Here's the drawing with two shaded views (mm, measured from the low corner). I have some questions. A direction names the side the tool comes from. Round coordinates to 2 decimals unless told otherwise and drop trailing zeros. Loops run counter-clockwise (first coordinate to the right, second up) from the corner with the lowest first, then second, coordinate; pieces in that order, holes last.
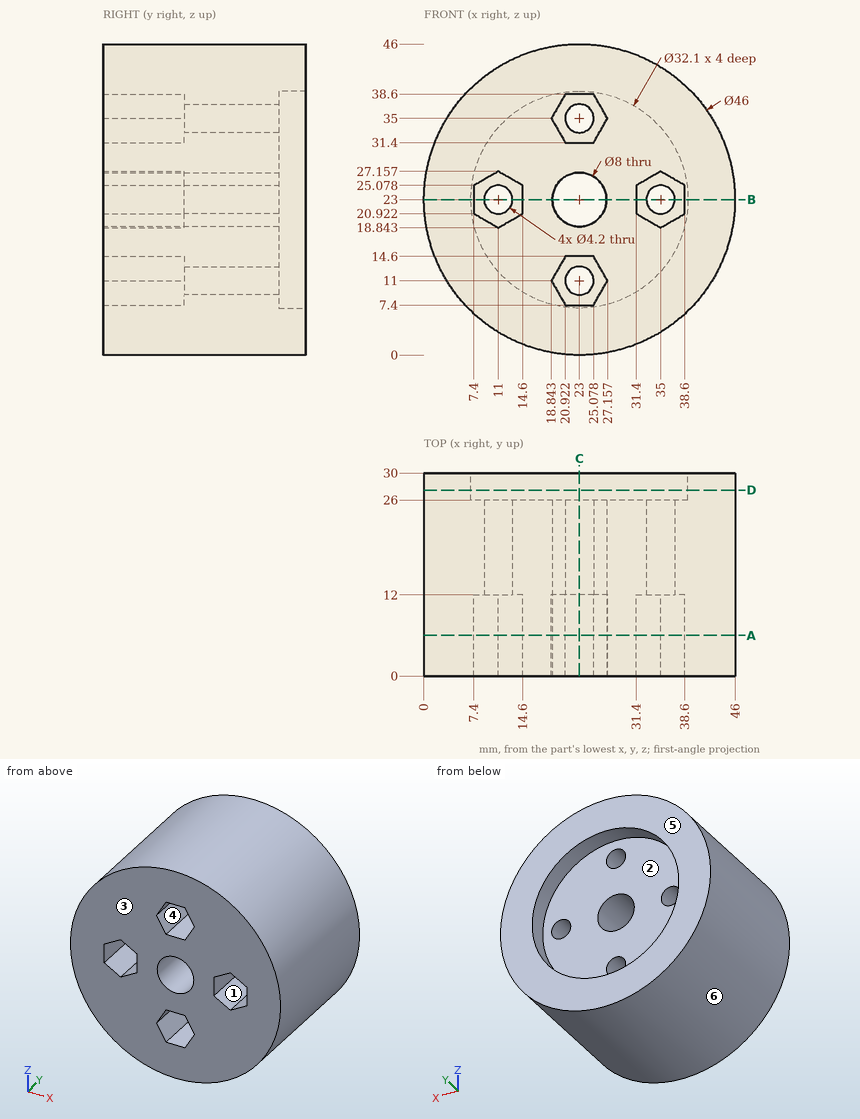
Item 1: If I drill on line 1 along X through (y, z) = (21, 23); line 2 along Z through (x, y) = (25, 1.5) (1 decimal); line 3 along Y through (x, z) = (21, 9.5), over which ranges is the centre line in solid material (lowest first)?
Results list:
line 1: x = 0 to 8.9, 13.1 to 19, 27 to 32.9, 37.1 to 46
line 2: z = 0.1 to 7.4, 14.6 to 19.5, 26.5 to 31.4, 38.6 to 45.9
line 3: y = 12 to 26
Item 2: Will these pins go through, and if not, where does the flat tip stop? pin 1 (6.5 mm diameter, centred on x = 11, z = 23, fed in from -Y); pin 2 (12 mm diameter, centred on y = 23.5, z = 10.5, fed in from +X); pin 3 (3.5 mm diameter, centred on y = 8, z = 22.5, fed in from -X).
Results list:
pin 1: stops at y = 12
pin 2: stops at x = 45.06
pin 3: stops at x = 0
Item 3: For the marked faces 1, 2 and 3, which set-ups out of +Z, -Z, +X, -X, +Y, -Y let a thin tool reach every point of the face, with its end or its side?
Results list:
face 1: -Y
face 2: +Y
face 3: +Z, -Z, +X, -X, -Y
Item 4: If we section it at D-D, the plane y = 27.5: Please give me the cut outline in (x, z).
Results list:
outline: circle Ø46 at (23, 23); hole circle Ø32.1 at (23, 23)
Item 5: If we section it at B-B, the plane z = 23: Please give me the cut outline in (x, y).
Results list:
outline: (0, 0) - (7.4, 0) - (7.4, 12) - (8.9, 12) - (8.9, 26) - (6.95, 26) - (6.95, 30) - (0, 30) - close; (13.1, 12) - (14.6, 12) - (14.6, 0) - (19, 0) - (19, 26) - (13.1, 26) - close; (27, 0) - (31.4, 0) - (31.4, 12) - (32.9, 12) - (32.9, 26) - (27, 26) - close; (37.1, 12) - (38.6, 12) - (38.6, 0) - (46, 0) - (46, 30) - (39.05, 30) - (39.05, 26) - (37.1, 26) - close
Item 6: We'd pull the mould along X, two halves only. Please class the marked faces 4, 5 and 6: released by +X, released by -X, zero draft, split by the parting line, or undercut.
Results list:
face 4: undercut
face 5: zero draft
face 6: split by the parting line
Item 7: If we section it at C-C, the plane x = 23: Please give me the cut outline in (y, z), then the cut area to 3 significant figures.
Results list:
outline: (0, 0) - (30, 0) - (30, 6.95) - (26, 6.95) - (26, 8.9) - (12, 8.9) - (12, 7.4) - (0, 7.4) - close; (0, 14.6) - (12, 14.6) - (12, 13.1) - (26, 13.1) - (26, 19) - (0, 19) - close; (0, 27) - (26, 27) - (26, 32.9) - (12, 32.9) - (12, 31.4) - (0, 31.4) - close; (0, 38.6) - (12, 38.6) - (12, 37.1) - (26, 37.1) - (26, 39.05) - (30, 39.05) - (30, 46) - (0, 46) - close
area: 753 mm2
Item 8: If we section it at A-A, the plane y = 6: Please give me the cut outline in (x, z).
Results list:
outline: circle Ø46 at (23, 23); hole (7.4, 20.92) - (11, 18.84) - (14.6, 20.92) - (14.6, 25.08) - (11, 27.16) - (7.4, 25.08) - close; hole (18.84, 11) - (20.92, 7.4) - (25.08, 7.4) - (27.16, 11) - (25.08, 14.6) - (20.92, 14.6) - close; hole (18.84, 35) - (20.92, 31.4) - (25.08, 31.4) - (27.16, 35) - (25.08, 38.6) - (20.92, 38.6) - close; hole circle Ø8 at (23, 23); hole (31.4, 20.92) - (35, 18.84) - (38.6, 20.92) - (38.6, 25.08) - (35, 27.16) - (31.4, 25.08) - close
